from build123d import *

# Parameters (mm, degrees)
SKETCH1_W           = 60
SKETCH1_H           = 60
BOSS_EXTRUDE1_DEPTH = 10
SKETCH2_R           = 1.15
CUT_EXTRUDE1_DEPTH  = 44.588989435
SKETCH3_R           = 1.15
CUT_EXTRUDE2_DEPTH  = 8
SKETCH5_R           = 5.25
CUT_EXTRUDE4_DEPTH  = 6.5
SKETCH6_R           = 3.25
CUT_EXTRUDE5_DEPTH  = 43.921439864


with BuildPart() as part:
    # Sketch1 → Boss-Extrude1 (new body)
    with BuildSketch(Plane.XY):
        Rectangle(SKETCH1_W, SKETCH1_H)
    extrude(amount=BOSS_EXTRUDE1_DEPTH)

    # Sketch2 → Cut-Extrude1 (cut, through all)
    with BuildSketch(Plane.XY.offset(10)):
        with BuildLine():
            ThreePointArc((-25, 26.15), (-26.15, 25), (-25, 23.85))
            Line((-25, 23.85), (-25, 26.15))
        make_face()
        with BuildLine():
            Line((-25, 26.15), (-25, 23.85))
            ThreePointArc((-25, 23.85), (-24.186827202, 24.186827202), (-23.85, 25))
            ThreePointArc((-23.85, 25), (-24.186827202, 25.813172798), (-25, 26.15))
        make_face()
        with Locations((25, 25)):
            Circle(SKETCH2_R)
        with Locations((25, -25)):
            Circle(SKETCH2_R)
        with Locations((-25, -25)):
            Circle(SKETCH2_R)
    extrude(amount=-CUT_EXTRUDE1_DEPTH, mode=Mode.SUBTRACT)

    # Sketch3 → Cut-Extrude2 (cut)
    # profile 1 of 4: a face of its own
    with BuildSketch(Plane.XY.offset(10)):
        Polygon((-26.212435565, 22.9), (-23.787564435, 22.9), (-22.575128869, 25), (-23.787564435, 27.1), (-26.212435565, 27.1), (-27.424871131, 25), align=None)
        with Locations((-25, 25)):
            Circle(SKETCH3_R, mode=Mode.SUBTRACT)
    # profile 2 of 4: a face of its own
    with BuildSketch(Plane.XY.offset(10)):
        Polygon((22.575128869, 25), (23.787564435, 27.1), (26.212435565, 27.1), (27.424871131, 25), (26.212435565, 22.9), (23.787564435, 22.9), align=None)
        with Locations((25, 25)):
            Circle(SKETCH3_R, mode=Mode.SUBTRACT)
    # profile 3 of 4: a face of its own
    with BuildSketch(Plane.XY.offset(10)):
        Polygon((26.212435565, -22.9), (23.787564435, -22.9), (22.575128869, -25), (23.787564435, -27.1), (26.212435565, -27.1), (27.424871131, -25), align=None)
        with Locations((25, -25)):
            Circle(SKETCH3_R, mode=Mode.SUBTRACT)
    # profile 4 of 4: a face of its own
    with BuildSketch(Plane.XY.offset(10)):
        Polygon((-22.575128869, -25), (-23.787564435, -27.1), (-26.212435565, -27.1), (-27.424871131, -25), (-26.212435565, -22.9), (-23.787564435, -22.9), align=None)
        with Locations((-25, -25)):
            Circle(SKETCH3_R, mode=Mode.SUBTRACT)
    extrude(amount=-CUT_EXTRUDE2_DEPTH, mode=Mode.SUBTRACT)

    # Sketch5 → Cut-Extrude4 (cut)
    with BuildSketch(Plane(origin=(0, 0, 0), x_dir=(-1, 0, 0), z_dir=(0, 0, -1))):
        with Locations((-12.5, 12.5)):
            Circle(SKETCH5_R)
        with Locations((12.5, 12.5)):
            Circle(SKETCH5_R)
        Circle(SKETCH5_R)
        with Locations((-12.5, -12.5)):
            Circle(SKETCH5_R)
        with Locations((12.5, -12.5)):
            Circle(SKETCH5_R)
    extrude(amount=-CUT_EXTRUDE4_DEPTH, mode=Mode.SUBTRACT)

    # Sketch6 → Cut-Extrude5 (cut, through all)
    with BuildSketch(Plane(origin=(0, 0, 6.5), x_dir=(-1, 0, 0), z_dir=(0, 0, -1))):
        with Locations((-12.5, 12.5)):
            Circle(SKETCH6_R)
        with Locations((12.5, 12.5)):
            Circle(SKETCH6_R)
        Circle(SKETCH6_R)
        with Locations((-12.5, -12.5)):
            Circle(SKETCH6_R)
        with Locations((12.5, -12.5)):
            Circle(SKETCH6_R)
    extrude(amount=-CUT_EXTRUDE5_DEPTH, mode=Mode.SUBTRACT)


solid = part.part
Geometry: final body of the model. Coordinates: model frame, mm. A direction names the side the tool comes from. Round coordinates to 2 decimals unless told otherwise and drop trailing zeros. Loops run counter-clockwise (first coordinate to the right, second up) from the corner with the lowest first, then second, coordinate; pieces in that order, holes last.
Q1. Access query for faces 1 (the flat face through (15, -15, 6.5)), 2 (the cylindrical face through (-9.253, 12.643, 8.226)), 3 (the flat face through (-26.81, 26.065, 6.056)). Directions: +Z, -Z, +X, -X, +Y, -Y. A direction counts if a zero-diameter tool reaches every point of the face in a straight line with its end or side. Return the directions, or none.
Q2. Pull-direction query (X, two-part tool) for faces 4 (the flat face through (-25, 27.1, 6)), 5 (the flat face through (0, 30, 5)), 6 (the flat face through (30, 0, 5)); classes: released by +X, released by -X, zero draft, split by the parting line, or undercut.
Q3. Pin query (flat end, axial travel): P1, Ø3.5, axis at x = 25, y = -25, coming from the +Z side; P2, Ø5, axis at x = -2.5, y = 0, coming from the -Z side. Return the tip coordinate at first contact, or that it passes through.
Q4. Section D-D on y = 12.5. Return loops of the section in (x, z).
Q5. Section C-C on z = 7.25. State how many separate pieces and enclosed holes the cut face has, plus the area to 3 significant figures.
Q6. Section A-A on x = 25. Return loops of the section in (y, z), plus the area to 3 significant figures.
Q7. Section B-B on y = 0. Return loops of the section in (x, z).
Q8. Material intervals for L1, parallel to Y at x = 12.5, z = 4.25; L2, parallel to Y at x = 25, z = 1.1; L3, parallel to X at y = 25.5, z = 3, sorted ascending.
Evaluation:
1. face 1: -Z
1. face 2: +Z, -Z
1. face 3: +Z
2. face 4: undercut
2. face 5: zero draft
2. face 6: released by +X
3. P1: stops at z = 2
3. P2: stops at z = 6.5
4. outline: (-30, 0) - (-17.75, 0) - (-17.75, 6.5) - (-15.75, 6.5) - (-15.75, 10) - (-30, 10) - close; (-9.25, 6.5) - (-7.25, 6.5) - (-7.25, 0) - (7.25, 0) - (7.25, 6.5) - (9.25, 6.5) - (9.25, 10) - (-9.25, 10) - close; (15.75, 6.5) - (17.75, 6.5) - (17.75, 0) - (30, 0) - (30, 10) - (15.75, 10) - close
5. separate pieces: 1
5. enclosed holes: 9
5. area: 3,370 mm2
6. outline: (-30, 0) - (-26.15, 0) - (-26.15, 2) - (-27.1, 2) - (-27.1, 10) - (-30, 10) - close; (-23.85, 0) - (23.85, 0) - (23.85, 2) - (22.9, 2) - (22.9, 10) - (-22.9, 10) - (-22.9, 2) - (-23.85, 2) - close; (26.15, 0) - (30, 0) - (30, 10) - (27.1, 10) - (27.1, 2) - (26.15, 2) - close
6. area: 524 mm2
7. outline: (-30, 0) - (-5.25, 0) - (-5.25, 6.5) - (-3.25, 6.5) - (-3.25, 10) - (-30, 10) - close; (3.25, 6.5) - (5.25, 6.5) - (5.25, 0) - (30, 0) - (30, 10) - (3.25, 10) - close
8. L1: y = -30 to -17.75, -7.25 to 7.25, 17.75 to 30
8. L2: y = -30 to -26.15, -23.85 to 23.85, 26.15 to 30
8. L3: x = -30 to -27.14, -22.86 to 22.86, 27.14 to 30
